Design review of the part shown in the three views and the two pictorial views. Dimensions are in mm from the part's minimum x, y and z. A direction names the side the tool comes from. Give positions to 0.01 mm unless a question says otherwise; leave off trailing zeros. Loops run counter-clockwise (first coordinate to the right, second up) from the corner with the lowest first, then second, coordinate; pieces in that order, holes last. Notation, with made-up numbers: (-23.5, -32.75) -> (28.5, -32.75) arc R28 cw to (28.5, 0.25) -> close; hole circle Ø11 at (49.25, -1.75). An arc over 180 degrees is marked (long way). Answer as CSV lines item,"result".
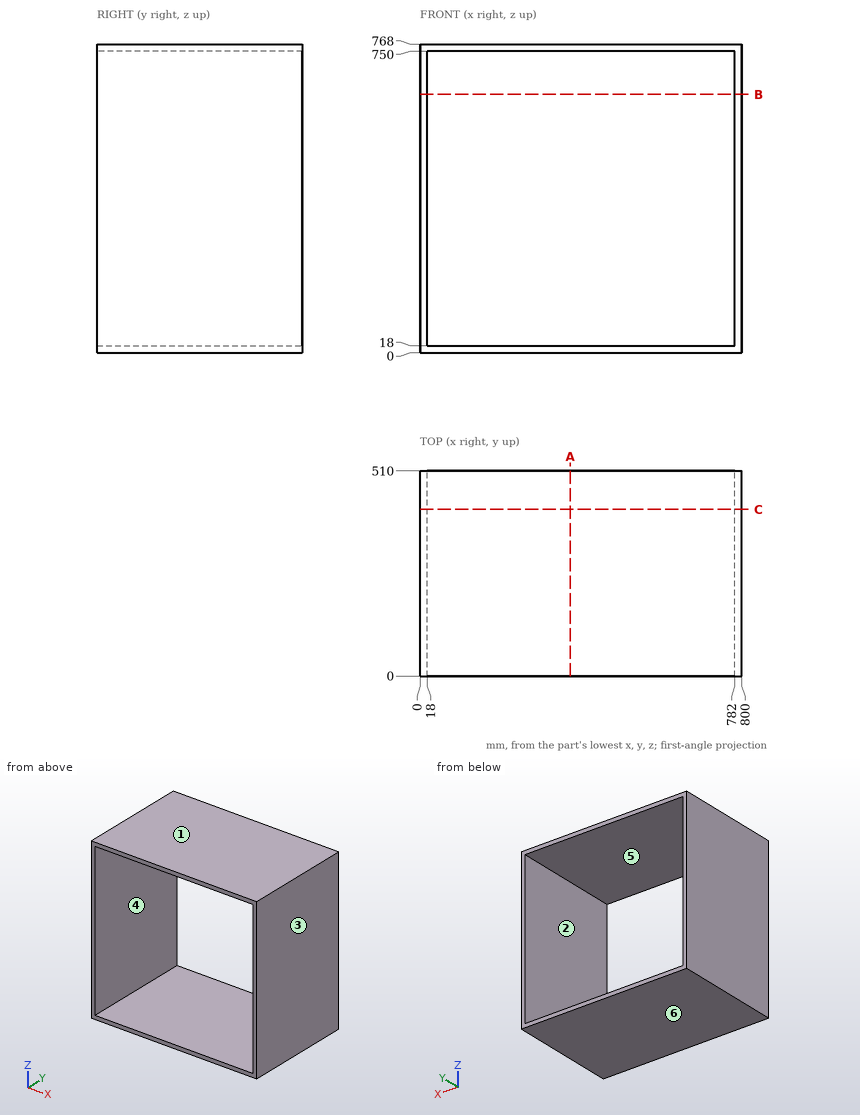
Q1. We need section A-A, the plane x = 373.5. State the section outline as (y, z) points, and give its area (3 significant figures).
Filled sheet:
outline,"(0, 0) -> (510, 0) -> (510, 18) -> (0, 18) -> close; (0, 750) -> (510, 750) -> (510, 768) -> (0, 768) -> close"
area,"18,400 mm^2"
Q2. To check wall thickness, follow probe 1 along Z at (x, y) = (610.5, 294.5); probe 2 along X at (y, z) = (88.5, 450). State the ranges of each line that lie inside material, in increasing order. Write a range as from..to.
Filled sheet:
probe 1,"z = 0..18, 750..768"
probe 2,"x = 0..18, 782..800"
Q3. We need section C-C, the plane y = 414. State the section outline as (x, z) points, and give its area (3 significant figures).
Filled sheet:
outline,"(0, 0) -> (800, 0) -> (800, 768) -> (0, 768) -> close; hole (18, 18) -> (782, 18) -> (782, 750) -> (18, 750) -> close"
area,"55,200 mm^2"
Q4. For the marked faces 1 and 2, list the 3-axis set-ups (+Z, -Z, +X, -X, +Y, -Y) from which the entire face can be reached by the end or side of a thin tool; tool diameter is ignored.
Filled sheet:
face 1,"+Z, +X, -X, +Y, -Y"
face 2,"+Y, -Y"
Q5. We need section B-B, the plane z = 643. State the section outline as (x, y) points, and give its area (3 significant figures).
Filled sheet:
outline,"(0, 0) -> (18, 0) -> (18, 510) -> (0, 510) -> close; (782, 0) -> (800, 0) -> (800, 510) -> (782, 510) -> close"
area,"18,400 mm^2"
Q6. The part is to be moulded in two halves that separate along Z. For the marked faces 3, 4, 5 and 6, say which applies: pulls with the +Z half, pulls with the -Z half, needs draft (parallel to the pull), parting line crosses it, or undercut.
Filled sheet:
face 3,"needs draft"
face 4,"undercut"
face 5,"undercut"
face 6,"pulls with the -Z half"
